from build123d import *

# Parameters (mm, degrees)
BOSS_EXTRUDE1_DEPTH = 2
SKETCH7_R           = 3.4
BOSS_EXTRUDE2_DEPTH = 1
CUT_EXTRUDE3_DEPTH  = 4


with BuildPart() as part:
    # Sketch2 → Boss-Extrude1 (new body)
    with BuildSketch(Plane.XY):
        with BuildLine():
            Line((10, -4.8), (10, 4.8))
            Line((10, 4.8), (0, 6))
            ThreePointArc((0, 6), (-6, 0), (0, -6))
            Line((0, -6), (10, -4.8))
        make_face()
    extrude(amount=BOSS_EXTRUDE1_DEPTH)

    # Sketch7 → Boss-Extrude2 (add)
    with BuildSketch(Plane.XY.offset(2)):
        Circle(SKETCH7_R)
    extrude(amount=BOSS_EXTRUDE2_DEPTH)

    # Sketch8 → Cut-Extrude3 (cut, through all)
    with BuildSketch(Plane.XY.offset(3)):
        with BuildLine():
            Line((-1, 1.122930178), (-1, -1.122930178))
            ThreePointArc((-1, -1.122930178), (1.503652947, 0), (-1, 1.122930178))
        make_face()
    extrude(amount=-CUT_EXTRUDE3_DEPTH, mode=Mode.SUBTRACT)


solid = part.part
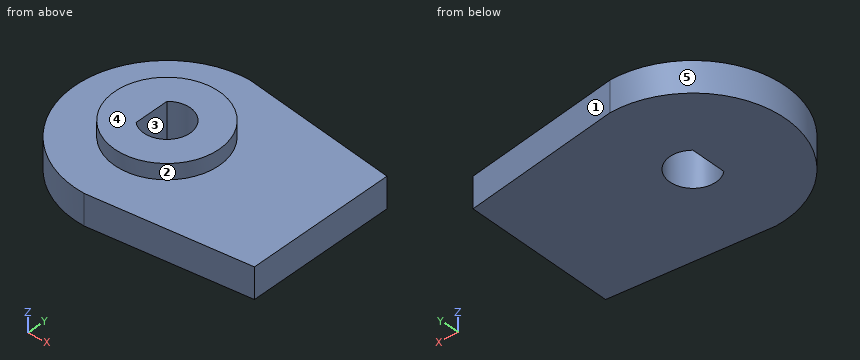
Geometry check sheet. Reference: the model listing, model coordinates, mm. Face numbers are marked on the shaded views. A direction names the side the tool comes from. Round coordinates to 2 decimals unless told otherwise and drop trailing zeros. Loops run counter-clockwise (first coordinate to the right, second up) from the corner with the lowest first, then second, coordinate; pieces in that order, holes last. Notation, with made-up numbers: (-11.75, -19.75) - (5.25, -19.75) arc R18 ccw to (5.25, -0.75) - close; hole circle Ø7 at (-29, -9). An arc over 180 degrees is marked (long way). Answer as CSV lines item,"result".
(1) Set-up check for the marked faces 1 and 2: record each of +Z, -Z, +X, -X, +Y, -Y from which the full face is reachable in a straight line by a thin tool's end or side.
Output values:
face 1,"+Z, -Z, +X, +Y"
face 2,"+Z"
(2) Material ranges on line 1 along Y through (x, z) = (0, 2.3); line 2 along X through (y, z) = (0, 0.8); line 3 along Z through (x, y) = (2.75, 4.75), recorded low to high.
Output values:
line 1,"y = -3.4 to -1.5, 1.5 to 3.4"
line 2,"x = -6 to -1, 1.5 to 10"
line 3,"z = 0 to 2"
(3) Cross-section at A-A, the plane y = 0. Enter the section's corners in (x, z), and give its area (3 significant figures).
Output values:
outline,"(-6, 0) - (-1, 0) - (-1, 3) - (-3.4, 3) - (-3.4, 2) - (-6, 2) - close; (1.5, 0) - (10, 0) - (10, 2) - (3.4, 2) - (3.4, 3) - (1.5, 3) - close"
area,"31.3 mm²"
(4) Release check for a two-part mould opening along X. For the marked faces 3, 4 and 5 record: released by +X, released by -X, zero draft, split by the parting line, or undercut.
Output values:
face 3,"undercut"
face 4,"zero draft"
face 5,"released by -X"
(5) Depth check by flat-ended pin: pin 1 Ø1.5 at (y, z) = (2.5, 2) entering from -X; pin 2 Ø1.5 at (x, y) = (5.5, 2.5) entering from -Z; pin 3 Ø1.5 at (x, z) = (7.5, 1.5) entering from -Y. Enter the tip coordinate at first touch or a pass-through.
Output values:
pin 1,"stops at x = -5.74"
pin 2,"stops at z = 0"
pin 3,"stops at y = -5.19"
(6) Cross-section at D-D, the plane y = 2.75. Enter the section's corners in (x, z).
Output values:
outline,"(-5.33, 0) - (10, 0) - (10, 2) - (2, 2) - (2, 3) - (-2, 3) - (-2, 2) - (-5.33, 2) - close"
(7) Cross-section at B-B, the plane z = 1.3. Enter the section's corners in (x, y), and give its area (3 significant figures).
Output values:
outline,"(0, -6) - (10, -4.8) - (10, 4.8) - (0, 6) arc R6 ccw to start; hole (-1, -1.12) arc R1.5 ccw (long way) to (-1, 1.12) - close"
area,"158 mm²"
(8) Cross-section at C-C, the plane x = 0.25. Enter the section's corners in (y, z), and give its area (3 significant figures).
Output values:
outline,"(-5.97, 0) - (-1.48, 0) - (-1.48, 3) - (-3.39, 3) - (-3.39, 2) - (-5.97, 2) - close; (1.48, 0) - (5.97, 0) - (5.97, 2) - (3.39, 2) - (3.39, 3) - (1.48, 3) - close"
area,"21.8 mm²"
